Here's how the part is built. I have some questions about the finished solid (model axes, mm). A direction names the side the tool comes from. Round coordinates to 2 decimals unless told otherwise and drop trailing zeros. Write each loop counter-clockwise with the first axis right and the second up, starting at its lowest first coordinate (ties: lowest second). Pieces come first, ordered by that corner, then holes. Notation, with made-up numbers: (-18, 32.5) -> (0, 32.5) arc R28 cw to (0, 69.5) -> close; hole circle Ø1 at (0.5, 69.5). An arc over 180 degrees is marked (long way). Answer as CSV lines item,"result".
from build123d import *

# Parameters (mm, degrees)
CROQUIS2_R                 = 4.7625
CORTAR_EXTRUIR1_DEPTH      = 41
CROQUIS3_R                 = 3.175
CORTAR_EXTRUIR2_DEPTH      = 61
CORTAR_EXTRUIR2_DEPTH_BACK = 61
CROQUIS4_R                 = 4.7625
CORTAR_EXTRUIR4_DEPTH      = 1.0000001
CORTAR_EXTRUIR4_DEPTH_BACK = 41.0000001


with BuildPart() as part:
    # Croquis1 → Revolución1 (revolve)
    with BuildSketch(Plane.XY):
        Polygon((0, 40), (60, 40), (60, 0), (55, 0), (55, 35), (0, 35), align=None)
    revolve(axis=Axis((0, 0, 0), (0, 1, 0)))

    # Croquis2 → Cortar-Extruir1 (cut, through all)
    with BuildSketch(Plane(origin=(0, 40, 0), x_dir=(1, 0, 0), z_dir=(0, 1, 0))):
        Circle(CROQUIS2_R)
    extrude(amount=-CORTAR_EXTRUIR1_DEPTH, mode=Mode.SUBTRACT)

    # Croquis3 → Cortar-Extruir2 (cut, two sides)
    with BuildSketch(Plane.XY) as cortar_extruir2_sk:
        with Locations((-10, 15)):
            Circle(CROQUIS3_R)
        with Locations((10, 15)):
            Circle(CROQUIS3_R)
    extrude(amount=CORTAR_EXTRUIR2_DEPTH, mode=Mode.SUBTRACT)
    extrude(cortar_extruir2_sk.sketch, amount=-CORTAR_EXTRUIR2_DEPTH_BACK, mode=Mode.SUBTRACT)

    # Croquis4 → Cortar-Extruir4 (cut, two sides)
    with BuildSketch(Plane(origin=(0, 40, 0), x_dir=(1, 0, 0), z_dir=(0, 1, 0))) as cortar_extruir4_sk:
        with Locations((0, 50)):
            Circle(CROQUIS4_R)
        with Locations((43.301270189, -25)):
            Circle(CROQUIS4_R)
        with Locations((-43.301270189, -25)):
            Circle(CROQUIS4_R)
    extrude(amount=CORTAR_EXTRUIR4_DEPTH, mode=Mode.SUBTRACT)
    extrude(cortar_extruir4_sk.sketch, amount=-CORTAR_EXTRUIR4_DEPTH_BACK, mode=Mode.SUBTRACT)


solid = part.part
Item 1: Suppose I cut it at A-A, the plane x = 0. List the corners of the cut face in (y, z) for me, then the cut area to 3 significant figures.
Results found:
outline,"(0, -60) -> (40, -60) -> (40, -54.76) -> (35, -54.76) -> (35, -55) -> (0, -55) -> close; (0, 55) -> (35, 55) -> (35, 4.76) -> (40, 4.76) -> (40, 60) -> (0, 60) -> close; (35, -45.24) -> (40, -45.24) -> (40, -4.76) -> (35, -4.76) -> close"
area,"855 mm²"
Item 2: For faces 5 (the flat face through (26, 0, 49)), 6 (the flat face through (-1, 35, 11)), which set-ups out of +Z, -Z, +X, -X, +Y, -Y let a thin tool reach every point of the face, with its end or its side?
Results found:
face 5,"+Z, -Z, +X, -X, -Y"
face 6,"-Y"
Item 3: Suppose I cut it at D-D, the plane y = 37. List the corners of the cut face in (x, z) for me (1 decimal), then the cut area to 3 significant figures.
Results found:
outline,"circle Ø120 at (0, 0); hole circle Ø9.5 at (-43.3, 25); hole circle Ø9.5 at (0, -50); hole circle Ø9.5 at (0, 0); hole circle Ø9.5 at (43.3, 25)"
area,"11,000 mm²"
Item 4: If we mould it in two halves opening along X, with no side actions, what happens to faces 1 (the flat face through (-12, 40, -1)), 2 (the cylindrical face through (50.806, 17.745, 21.065)), 3 (the cylindrical face through (-3.78, 37.53, 2.9)), 4 (the cylindrical face through (55.425, 19.72, 22.98))? For each: pulls with the +X half, pulls with the -X half, needs draft (parallel to the pull), parting line crosses it, or undercut.
Results found:
face 1,"needs draft"
face 2,"undercut"
face 3,"undercut"
face 4,"parting line crosses it"
Item 5: Suppose I cut it at C-C, the plane y = 15. List the corners of the cut face in (x, z) for me (3 decimals), then the cut area to 3 significant figures.
Results found:
outline,"(-13.175, -58.536) -> (-13.175, -53.399) arc R55 cw to (-13.175, 53.399) -> (-13.175, 58.536) arc R60 ccw to start; (-6.825, -59.611) arc R60 ccw to (6.825, -59.611) -> (6.825, -54.575) arc R55 cw to (-6.825, -54.575) -> close; (-6.825, 54.575) arc R55 cw to (6.825, 54.575) -> (6.825, 59.611) arc R60 ccw to (-6.825, 59.611) -> close; (13.175, -58.536) arc R60 ccw to (13.175, 58.536) -> (13.175, 53.399) arc R55 cw to (13.175, -53.399) -> close"
area,"1,680 mm²"
Item 6: Suppose I cut it at B-B, the plane z = 0. List the corners of the cut face in (x, y) for me.
Results found:
outline,"(-60, 0) -> (-55, 0) -> (-55, 35) -> (-4.76, 35) -> (-4.76, 40) -> (-60, 40) -> close; (4.76, 35) -> (55, 35) -> (55, 0) -> (60, 0) -> (60, 40) -> (4.76, 40) -> close"
Item 7: I need wall thicknesses on L1, parallel to Y at x = 10, z = 57.5 (3 decimals); L2, parallel to X at y = 38, z = 25; L3, parallel to Z at x = 20, y = 31. Which ranges of each line are inside material? Lowest first, please.
Results found:
L1,"y = 0 to 11.825, 18.175 to 40"
L2,"x = -54.54 to -48.06, -38.54 to 38.54, 48.06 to 54.54"
L3,"z = -56.57 to -51.23, 51.23 to 56.57"
Item 8: Will these pins go through, and if not, where does the flat tip stop? pin 1 (7.5 mm diameter, centred on x = 0, z = -50, fed in from -Y); pin 2 (5 mm diameter, centred on x = -36, z = -1.5, fed in from -Y); pin 3 (4 mm diameter, centred on y = 15.5, z = 40.5, fed in from -X); pin 4 (7.5 mm diameter, centred on x = -10, y = 15, fed in from +Z).
Results found:
pin 1,"passes through"
pin 2,"stops at y = 35"
pin 3,"stops at x = -46.02"
pin 4,"stops at z = 59.67"
